```python
from build123d import *

# Parameters (mm, degrees)
SKETCH1_R           = 3.175
SKETCH1_R_2         = 3.001746658
BOSS_EXTRUDE1_DEPTH = 12.7
SKETCH6_R           = 3.3734375
CUT_EXTRUDE6_DEPTH  = 12.7
SKETCH6_3_R         = 5.55625
SKETCH6_3_R_2       = 3.3734375
CUT_EXTRUDE7_DEPTH  = 6.35
CUT_EXTRUDE8_DEPTH  = 6.35
SKETCH7_W           = 101.6
SKETCH7_H           = 27.94
CUT_EXTRUDE9_DEPTH  = 12.7
SKETCH8_R           = 3.3734375
CUT_EXTRUDE10_DEPTH = 12.7
SKETCH8_3_R         = 5.55625
SKETCH8_3_R_2       = 3.3734375
CUT_EXTRUDE11_DEPTH = 6.35


with BuildPart() as part:
    # Sketch1 → Boss-Extrude1 (new body)
    with BuildSketch(Plane.XY):
        Polygon((0, 152.4), (0, 0), (63.5, 0), (63.5, 50.8), (215.9, 50.8), (215.9, -76.2), (285.75, -76.2), (285.75, 152.4), align=None)
        with Locations((19.05, 12.7)):
            Circle(SKETCH1_R, mode=Mode.SUBTRACT)
        with Locations((19.05, 38.1)):
            Circle(SKETCH1_R, mode=Mode.SUBTRACT)
        with Locations((44.45, 12.7)):
            Circle(SKETCH1_R, mode=Mode.SUBTRACT)
        with Locations((44.45, 38.1)):
            Circle(SKETCH1_R, mode=Mode.SUBTRACT)
        with Locations((247.65, -63.5)):
            Circle(SKETCH1_R, mode=Mode.SUBTRACT)
        with Locations((273.05, -63.5)):
            Circle(SKETCH1_R, mode=Mode.SUBTRACT)
        with Locations((247.65, -38.1)):
            Circle(SKETCH1_R, mode=Mode.SUBTRACT)
        with Locations((273.05, -38.1)):
            Circle(SKETCH1_R, mode=Mode.SUBTRACT)
        with Locations((247.65, -12.7)):
            Circle(SKETCH1_R, mode=Mode.SUBTRACT)
        with Locations((247.65, 12.7)):
            Circle(SKETCH1_R, mode=Mode.SUBTRACT)
        with Locations((247.65, 38.1)):
            Circle(SKETCH1_R, mode=Mode.SUBTRACT)
        with Locations((44.45, 63.5)):
            Circle(SKETCH1_R, mode=Mode.SUBTRACT)
        with Locations((69.85, 63.5)):
            Circle(SKETCH1_R, mode=Mode.SUBTRACT)
        with Locations((44.45, 88.9)):
            Circle(SKETCH1_R, mode=Mode.SUBTRACT)
        with Locations((69.85, 88.9)):
            Circle(SKETCH1_R, mode=Mode.SUBTRACT)
        with Locations((95.25, 63.5)):
            Circle(SKETCH1_R, mode=Mode.SUBTRACT)
        with Locations((120.65, 63.5)):
            Circle(SKETCH1_R, mode=Mode.SUBTRACT)
        with Locations((95.25, 88.9)):
            Circle(SKETCH1_R, mode=Mode.SUBTRACT)
        with Locations((120.65, 88.9)):
            Circle(SKETCH1_R, mode=Mode.SUBTRACT)
        with Locations((19.05, 114.3)):
            Circle(SKETCH1_R, mode=Mode.SUBTRACT)
        with Locations((44.45, 114.3)):
            Circle(SKETCH1_R, mode=Mode.SUBTRACT)
        with Locations((69.85, 114.3)):
            Circle(SKETCH1_R, mode=Mode.SUBTRACT)
        with Locations((19.05, 139.7)):
            Circle(SKETCH1_R, mode=Mode.SUBTRACT)
        with Locations((44.45, 139.7)):
            Circle(SKETCH1_R, mode=Mode.SUBTRACT)
        with Locations((69.85, 139.7)):
            Circle(SKETCH1_R, mode=Mode.SUBTRACT)
        with Locations((95.25, 114.3)):
            Circle(SKETCH1_R, mode=Mode.SUBTRACT)
        with Locations((120.65, 114.3)):
            Circle(SKETCH1_R, mode=Mode.SUBTRACT)
        with Locations((95.25, 139.7)):
            Circle(SKETCH1_R, mode=Mode.SUBTRACT)
        with Locations((120.65, 139.7)):
            Circle(SKETCH1_R, mode=Mode.SUBTRACT)
        with Locations((146.05, 63.5)):
            Circle(SKETCH1_R, mode=Mode.SUBTRACT)
        with Locations((171.45, 63.5)):
            Circle(SKETCH1_R, mode=Mode.SUBTRACT)
        with Locations((196.85, 63.5)):
            Circle(SKETCH1_R, mode=Mode.SUBTRACT)
        with Locations((146.05, 88.9)):
            Circle(SKETCH1_R, mode=Mode.SUBTRACT)
        with Locations((171.45, 88.9)):
            Circle(SKETCH1_R, mode=Mode.SUBTRACT)
        with Locations((196.85, 88.9)):
            Circle(SKETCH1_R, mode=Mode.SUBTRACT)
        with Locations((222.25, 63.5)):
            Circle(SKETCH1_R, mode=Mode.SUBTRACT)
        with Locations((247.65, 63.5)):
            Circle(SKETCH1_R, mode=Mode.SUBTRACT)
        with Locations((273.05, 63.5)):
            Circle(SKETCH1_R, mode=Mode.SUBTRACT)
        with Locations((222.25, 88.9)):
            Circle(SKETCH1_R, mode=Mode.SUBTRACT)
        with Locations((247.65, 88.9)):
            Circle(SKETCH1_R, mode=Mode.SUBTRACT)
        with Locations((273.05, 88.9)):
            Circle(SKETCH1_R, mode=Mode.SUBTRACT)
        with Locations((146.05, 114.3)):
            Circle(SKETCH1_R, mode=Mode.SUBTRACT)
        with Locations((171.45, 114.3)):
            Circle(SKETCH1_R, mode=Mode.SUBTRACT)
        with Locations((196.85, 114.3)):
            Circle(SKETCH1_R, mode=Mode.SUBTRACT)
        with Locations((146.05, 139.7)):
            Circle(SKETCH1_R, mode=Mode.SUBTRACT)
        with Locations((171.45, 139.7)):
            Circle(SKETCH1_R, mode=Mode.SUBTRACT)
        with Locations((196.85, 139.7)):
            Circle(SKETCH1_R, mode=Mode.SUBTRACT)
        with Locations((222.25, 114.3)):
            Circle(SKETCH1_R, mode=Mode.SUBTRACT)
        with Locations((247.65, 114.3)):
            Circle(SKETCH1_R, mode=Mode.SUBTRACT)
        with Locations((273.05, 114.3)):
            Circle(SKETCH1_R, mode=Mode.SUBTRACT)
        with Locations((222.25, 139.7)):
            Circle(SKETCH1_R, mode=Mode.SUBTRACT)
        with Locations((247.65, 139.7)):
            Circle(SKETCH1_R, mode=Mode.SUBTRACT)
        with Locations((273.05, 139.7)):
            Circle(SKETCH1_R, mode=Mode.SUBTRACT)
        with Locations((273.05, 38.1)):
            Circle(SKETCH1_R_2, mode=Mode.SUBTRACT)
    extrude(amount=BOSS_EXTRUDE1_DEPTH)

    # Sketch6 → Cut-Extrude6 (cut)
    with BuildSketch(Plane.XY.offset(12.7)):
        with Locations((23.114, 60.1472)):
            Circle(SKETCH6_R)
        with Locations((23.114, 85.5472)):
            Circle(SKETCH6_R)
    extrude(amount=-CUT_EXTRUDE6_DEPTH, mode=Mode.SUBTRACT)

    # Sketch6<3> → Cut-Extrude7 (cut)
    # profile 1 of 2: a face of its own
    with BuildSketch(Plane.XY.offset(12.7)):
        with Locations((23.114, 85.5472)):
            Circle(SKETCH6_3_R)
        with Locations((23.114, 85.5472)):
            Circle(SKETCH6_3_R_2, mode=Mode.SUBTRACT)
    # profile 2 of 2: a face of its own
    with BuildSketch(Plane.XY.offset(12.7)):
        with BuildLine():
            Line((23.114, 56.7737625), (23.114, 54.59095))
            ThreePointArc((23.114, 54.59095), (27.042862053, 56.218337947), (28.67025, 60.1472))
            ThreePointArc((28.67025, 60.1472), (23.114, 65.70345), (17.55775, 60.1472))
            Line((17.55775, 60.1472), (19.7405625, 60.1472))
            ThreePointArc((19.7405625, 60.1472), (23.114, 63.5206375), (26.4874375, 60.1472))
            ThreePointArc((26.4874375, 60.1472), (25.499380532, 57.761819468), (23.114, 56.7737625))
        make_face()
    extrude(amount=-CUT_EXTRUDE7_DEPTH, mode=Mode.SUBTRACT)

    # Sketch6<4> → Cut-Extrude8 (cut)
    with BuildSketch(Plane.XY.offset(12.7)):
        with BuildLine():
            ThreePointArc((17.55775, 60.1472), (19.185137947, 56.218337947), (23.114, 54.59095))
            Line((23.114, 54.59095), (23.114, 56.7737625))
            ThreePointArc((23.114, 56.7737625), (20.728619468, 57.761819468), (19.7405625, 60.1472))
            Line((19.7405625, 60.1472), (17.55775, 60.1472))
        make_face()
        with BuildLine():
            Line((23.114, 56.7737625), (23.114, 54.59095))
            ThreePointArc((23.114, 54.59095), (27.042862053, 56.218337947), (28.67025, 60.1472))
            ThreePointArc((28.67025, 60.1472), (23.114, 65.70345), (17.55775, 60.1472))
            Line((17.55775, 60.1472), (19.7405625, 60.1472))
            ThreePointArc((19.7405625, 60.1472), (23.114, 63.5206375), (26.4874375, 60.1472))
            ThreePointArc((26.4874375, 60.1472), (25.499380532, 57.761819468), (23.114, 56.7737625))
        make_face()
    extrude(amount=-CUT_EXTRUDE8_DEPTH, mode=Mode.SUBTRACT)

    # Sketch7 → Cut-Extrude9 (cut)
    with BuildSketch(Plane.XY.offset(12.7)):
        with Locations((50.8, 138.43)):
            Rectangle(SKETCH7_W, SKETCH7_H)
    extrude(amount=-CUT_EXTRUDE9_DEPTH, mode=Mode.SUBTRACT)

    # Sketch8 → Cut-Extrude10 (cut)
    with BuildSketch(Plane.XY.offset(12.7)):
        with Locations((257.175, -22.1742)):
            Circle(SKETCH8_R)
        with Locations((257.175, 3.2258)):
            Circle(SKETCH8_R)
    extrude(amount=-CUT_EXTRUDE10_DEPTH, mode=Mode.SUBTRACT)

    # Sketch8<3> → Cut-Extrude11 (cut)
    # profile 1 of 2: a face of its own
    with BuildSketch(Plane.XY.offset(12.7)):
        with Locations((257.175, 3.2258)):
            Circle(SKETCH8_3_R)
        with Locations((257.175, 3.2258)):
            Circle(SKETCH8_3_R_2, mode=Mode.SUBTRACT)
    # profile 2 of 2: a face of its own
    with BuildSketch(Plane.XY.offset(12.7)):
        with Locations((257.175, -22.1742)):
            Circle(SKETCH8_3_R)
        with Locations((257.175, -22.1742)):
            Circle(SKETCH8_3_R_2, mode=Mode.SUBTRACT)
    extrude(amount=-CUT_EXTRUDE11_DEPTH, mode=Mode.SUBTRACT)


solid = part.part
```
The listing builds one solid part. Answer for the finished solid, in the listing's coordinates (mm). A direction names the side the tool comes from. Round coordinates to 2 decimals unless told otherwise and drop trailing zeros. Loops run counter-clockwise (first coordinate to the right, second up) from the corner with the lowest first, then second, coordinate; pieces in that order, holes last.
Q1. Find the intervals of material crossed by line 1 (X direction, y = 2.5, z = 12.25); line 2 (Y direction, x = 171.45, z = 3) (3 decimals); line 3 (Y direction, x = 196, z = 0.5), in increasing order.
Q2. Which of the six approach directions +Z, -Z, +X, -X, +Y, -Y give full straight-line access (tool end or side, diameter ignored) to faces 1 (the face through (260, 1, 6.35)), 2 (the face through (215.9, -12, 6)), 3 (the face through (123.68, 64.45, 6.26))?
Q3. Section C-C, the plane y = 12.7 is taken. Determine the outline of the cut face in (x, z) (3 decimals), then the cut area to 3 significant figures.
Q4. Section D-D, the plane x = 273.05 is taken. Count the separate pieces of the cut face and the enclosed holes in it, then the cut area to 3 significant figures.
Q5. Section A-A, the plane y = -12.7 is taken. Determine the outline of the cut face in (x, z) (3 decimals), then the cut area to 3 significant figures.
Q6. Given pin 1 Ø2 at (x, z) = (38.5, 10.5) entering from +Y; pin 2 Ø8.5 at (x, y) = (146.05, 114.3) entering from -Z; pin 3 Ø5.5 at (x, y) = (273.05, 139.7) entering from +Z; pin 4 Ø2 at (x, z) = (189.5, 10) entering from -Y, each flat-ended and moving along its own axis, determine where each tip first touches the part or whether it passes through.
Q7. For a pull along Y with two mould halves and no side action, classify faces 4 (the face through (0, 63, 6)), 5 (the face through (122.115, 86.083, 6.261)) as released by +Y, released by -Y, zero draft, split by the parting line, or undercut.
Q8. Section B-B, the plane x = 171.45 is taken. Determine the outline of the cut face in (y, z) (3 decimals), then the cut area to 3 significant figures.
Completed:
1. line 1: x = 0 to 63.5, 215.9 to 251.67, 262.68 to 285.75
1. line 2: y = 50.8 to 60.325, 66.675 to 85.725, 92.075 to 111.125, 117.475 to 136.525, 142.875 to 152.4
1. line 3: y = 50.8 to 60.44, 66.56 to 85.84, 91.96 to 111.24, 117.36 to 136.64, 142.76 to 152.4
2. face 1: +Z
2. face 2: +Z, -Z, -Y
2. face 3: +Z, -Z
3. outline: (0, 0) - (15.875, 0) - (15.875, 12.7) - (0, 12.7) - close; (22.225, 0) - (41.275, 0) - (41.275, 12.7) - (22.225, 12.7) - close; (47.625, 0) - (63.5, 0) - (63.5, 12.7) - (47.625, 12.7) - close; (215.9, 0) - (244.475, 0) - (244.475, 12.7) - (215.9, 12.7) - close; (250.825, 0) - (285.75, 0) - (285.75, 12.7) - (250.825, 12.7) - close
3. area: 1,450 mm2
4. separate pieces: 8
4. enclosed holes: 0
4. area: 2,340 mm2
5. outline: (215.9, 0) - (244.475, 0) - (244.475, 12.7) - (215.9, 12.7) - close; (250.825, 0) - (285.75, 0) - (285.75, 12.7) - (250.825, 12.7) - close
5. area: 806 mm2
6. pin 1: stops at y = 124.46
6. pin 2: stops at z = 0
6. pin 3: passes through
6. pin 4: stops at y = 50.8
7. face 4: zero draft
7. face 5: undercut
8. outline: (50.8, 0) - (60.325, 0) - (60.325, 12.7) - (50.8, 12.7) - close; (66.675, 0) - (85.725, 0) - (85.725, 12.7) - (66.675, 12.7) - close; (92.075, 0) - (111.125, 0) - (111.125, 12.7) - (92.075, 12.7) - close; (117.475, 0) - (136.525, 0) - (136.525, 12.7) - (117.475, 12.7) - close; (142.875, 0) - (152.4, 0) - (152.4, 12.7) - (142.875, 12.7) - close
8. area: 968 mm2
